from build123d import *

# Parameters (mm, degrees)
BOSS_EXTRUDE1_DEPTH                          = 20
FILLET1_R                                    = 1
FILLET2_R                                    = 4
CSK_FOR_M3_COUNTERSUNK_FLAT_HEAD_SCR_2_COUNT = 2
CSK_FOR_M3_COUNTERSUNK_FLAT_HEAD_SCR_2_PITCH = 10
CUT_REVOLVE1_ANGLE                           = 110
CUT_REVOLVE1_OTHER_WAY_ANGLE                 = 150


with BuildPart() as part:
    # Sketch1 → Boss-Extrude1 (new body)
    with BuildSketch(Plane(origin=(0, 0, 0), x_dir=(0, 0, -1), z_dir=(1, 0, 0))):
        with BuildLine():
            Line((-19.05, 43.688898834), (19.05, 43.688898834))
            Line((19.05, 43.688898834), (19.05, 41.688898834))
            Line((19.05, 41.688898834), (13.05, 35.688898834))
            ThreePointArc((13.05, 35.688898834), (22.67902305, 30.490357714), (30.427400447, 22.763420262))
            Line((30.427400447, 22.763420262), (37.355603678, 26.763420262))
            Line((37.355603678, 26.763420262), (38.855603678, 24.16534405))
            Line((38.855603678, 24.16534405), (29.533039808, 18.782959291))
            ThreePointArc((29.533039808, 18.782959291), (-30.310889132, -17.5), (31.033039808, 16.184883079))
            Line((31.033039808, 16.184883079), (40.355603678, 21.567267839))
            Line((40.355603678, 21.567267839), (41.855603678, 18.969191628))
            Line((41.855603678, 18.969191628), (34.927400447, 14.969191628))
            ThreePointArc((34.927400447, 14.969191628), (-15.065912825, -34.885788951), (-13.05, 35.688898834))
            Line((-13.05, 35.688898834), (-19.05, 41.688898834))
            Line((-19.05, 41.688898834), (-19.05, 43.688898834))
        make_face()
    extrude(amount=BOSS_EXTRUDE1_DEPTH)

    # Fillet1
    fillet1_edges = [part.edges().sort_by_distance(p)[0] for p in [
        (10, 35.688898834, 13.05),
        (10, 35.688898834, -13.05),
        (10, 22.763420262, -30.427400447),
        (10, 14.969191628, -34.927400447),
    ]]
    fillet(fillet1_edges, radius=FILLET1_R)

    # Fillet2
    fillet2_edges = [part.edges().sort_by_distance(p)[0] for p in [
        (10, 18.782959291, -29.533039808),
        (10, 16.184883079, -31.033039808),
    ]]
    fillet(fillet2_edges, radius=FILLET2_R)

    # Sketch3 → CSK for M3 Countersunk Flat Head Screw1 (revolve, cut)
    with BuildSketch(Plane(origin=(15, 16.969191628, -38.391502063), x_dir=(0, 0.49999999999999817, -0.8660254037844398), z_dir=(1, 0, 0))):
        Polygon((0, 0), (0, 61.335696254), (1.7, 61.335696254), (1.7, 1.45), (3.15, 0), align=None)
    csk_for_m3_countersunk_flat_head_screw1 = revolve(axis=Axis((15, 11.469930314, -41.566502063), (0, 0.8660254037844398, 0.4999999999999981)), mode=Mode.SUBTRACT)

    # CSK for M3 Countersunk Flat Head Scr 2: CSK for M3 Countersunk Flat Head Screw1 ×2
    with Locations(*[(-i * CSK_FOR_M3_COUNTERSUNK_FLAT_HEAD_SCR_2_PITCH, 0, 0) for i in range(1, CSK_FOR_M3_COUNTERSUNK_FLAT_HEAD_SCR_2_COUNT)]):
        add(csk_for_m3_countersunk_flat_head_screw1, mode=Mode.SUBTRACT)

    # Sketch4 → Cut-Revolve1 (revolve, cut)
    with BuildSketch(Plane.XY):
        with BuildLine():
            Line((-8.002699019, -33.015043362), (-8.002699019, -46))
            Line((-8.002699019, -46), (28, -46))
            Line((28, -46), (28, -33.01666204))
            ThreePointArc((28, -33.01666204), (9.998426404, -37.999999965), (-8.002699019, -33.015043362))
        make_face()
    revolve(axis=Axis((-3.558727933, 0, 0), (1, 0, 0)), revolution_arc=CUT_REVOLVE1_ANGLE, mode=Mode.SUBTRACT)

    # Sketch4 → Cut-Revolve1 other way (revolve, cut)
    with BuildSketch(Plane.XY):
        with BuildLine():
            Line((-8.002699019, -33.015043362), (-8.002699019, -46))
            Line((-8.002699019, -46), (28, -46))
            Line((28, -46), (28, -33.01666204))
            ThreePointArc((28, -33.01666204), (9.998426404, -37.999999965), (-8.002699019, -33.015043362))
        make_face()
    revolve(axis=Axis((-3.558727933, 0, 0), (-1, 0, 0)), revolution_arc=CUT_REVOLVE1_OTHER_WAY_ANGLE, mode=Mode.SUBTRACT)


solid = part.part
Design review of the part built by this model. Coordinates are the model's own, in mm. A direction names the side the tool comes from. Coordinates: 2 decimals unless noted, no trailing zeros. Loops run counter-clockwise (first coordinate to the right, second up) from the corner with the lowest first, then second, coordinate; pieces in that order, holes last.
Item 1: Add section A-A (z = -17.5). Give the number of separate pieces and of enclosed holes in the cut face, and give its area (3 significant figures).
Completed:
separate pieces: 3
enclosed holes: 0
area: 197 mm2
Item 2: Clearance check with flat-ended pins moving along their axes: pin 1 (1 mm diameter, centred on x = 5.5, z = -30.5, fed in from +Y); pin 2 (1.6 mm diameter, centred on x = 11.5, y = 42.5, fed in from +Z); pin 3 (10 mm diameter, centred on x = 12, z = -33.5, fed in from -Y); pin 4 (1 mm diameter, centred on y = -24.5, z = 22, fed in from +X). State where each tip first meets the part, or that it passes through.
Completed:
pin 1: stops at y = 23.34
pin 2: stops at z = 19.05
pin 3: stops at y = -25.06
pin 4: passes through
Item 3: For faces 1 (the flat face through (10, 43, -19.05)), 2 (the cylindrical face through (9.86, 34.085, 16.799)), 3 (the flat face through (20, 33.5, -11.5)), 4 (the flat face through (9.86, 39.27, -16.63)), 5 (the flat face through (9.9, 22.4, -35.8)), list the 3-axis set-ups (+Z, -Z, +X, -X, +Y, -Y) from which the entire face can be reached by the end or side of a thin tool; tool diameter is ignored.
Completed:
face 1: -Z, +X, -X, +Y
face 2: +Z, +X, -X
face 3: +Z, -Z, +X, +Y, -Y
face 4: -Z, +X, -X
face 5: +X, -X
Item 4: Wall thickness on L1, parallel to Z at x = 16.25, y = 21; L2, parallel to Y at x = 9, z = 0; L3, parallel to Y at x = 12.75, z = -23: over which ranges is each line inside the solid? List them lowest first.
Completed:
L1: z = -40.68 to -39.37, -33.37 to -28.12, 28 to 30.99
L2: y = -37.99 to -35, 35 to 43.69
L3: y = -30.11 to -26.38, 26.38 to 30.25
Item 5: Add section B-B (y = 39). Write out the cut boundary in (x, z).
Completed:
outline: (0, -16.36) - (20, -16.36) - (20, 16.36) - (0, 16.36) - close
Item 6: Draft analysis for pull direction Z (two halves, no side actions). For faces 6 (the flat face through (9.86, 25.483, -38.095)), 7 (the flat face through (10, 43, 19.05)), 8 (the cylindrical face through (3.57, 19.34, -38.08)), state which applies: pulls with the +Z half, pulls with the -Z half, needs draft (parallel to the pull), parting line crosses it, or undercut.
Completed:
face 6: pulls with the -Z half
face 7: pulls with the +Z half
face 8: undercut
